Source: CAD feature listing. Evaluate the final solid. Frame: model axes, mm. A direction names the side the tool comes from. Round coordinates to 2 decimals unless told otherwise and drop trailing zeros. Loops run counter-clockwise (first coordinate to the right, second up) from the corner with the lowest first, then second, coordinate; pieces in that order, holes last. Notation, with made-up numbers: (55.5, -3) - (113.5, -3) arc R18 ccw to (113.5, 29) - close; hole circle Ø3 at (-19, 65). An arc over 180 degrees is marked (long way). One line per question, with ' | ' between items. Start each with the question number.
1. Mould query, pull axis Z, two halves, no side actions, for faces 1 (the cylindrical face through (28.14, 71.59, -8.86)), 2 (the flat face through (27.41, 65, 11.34)), 3 (the flat face through (26, 63.5, 11)). Classes: pulls with the +Z half, pulls with the -Z half, needs draft (parallel to the pull), parting line crosses it, or undercut.
2. Pin query (flat end, axial travel): pin 1 (1.5 mm diameter, centred on x = 13, y = 61, fed in from +Z); pin 2 (6 mm diameter, centred on x = -11.5, y = 41.5, fed in from +Z); pin 3 (8 mm diameter, centred on x = 1.5, z = 5.5, fed in from +Y). Return the tip coordinate at first contact, or that it passes through.
3. Cut plane C-C (z = 0). Return loops of the section in (x, y), then the cut area to 3 significant figures.
4. Access query for faces 4 (the cylindrical face through (28.14, 32.07, 8.86)), 5 (the cylindrical face through (25.865, 70.648, -10.724)), 6 (the cylindrical face through (-4.036, 32.955, -30.736)). Directions: +Z, -Z, +X, -X, +Y, -Y. A direction counts if a zero-diameter tool reaches every point of the face in a straight line with its end or side. Return the directions, or none.
5. Ray query, line 1 (Y direction, x = 3, z = -28); line 2 (X direction, y = 30, z = 0). Return the intervals inside material, ascending.
6. Cut plane A-A (y = 12). Return loops of the section in (x, z).
7. Cut plane B-B (x = 0). Return loops of the section in (y, z), then the cut area to 3 significant figures.
Autodesk Inventor part; units mm, degrees
ref_plane "YZ Plane" through (0, 0, 0) normal (1, 0, 0) x (0, 1, 0)
ref_plane "XZ Plane" through (0, 0, 0) normal (0, 1, 0) x (-1, 0, 0)
ref_plane "XY Plane" through (0, 0, 0) normal (0, 0, 1) x (1, 0, 0)
sketch "Sketch1" plane through (0, 0, 0) normal (0, 0, 1) x (1, 0, 0)
  line L0 (0, 0) -> (31, 0)
  line L1 (31, 0) -> (31, 65)
  line L2 (31, 65) -> (29.5, 65)
  line L3 (29.5, 65) -> (29.5, 78)
  line L4 (29.5, 78) -> (28, 78)
  line L5 (28, 76.5) -> (28, 76.5)
  line L6 (28, 78) -> (28, 63.5)
  line L7 (28, 63.5) -> (29.5, 63.5)
  line L8 (29.5, 63.5) -> (29.5, 1.5)
  line L9 (29.5, 1.5) -> (0, 1.5)
  line L10 (0, 0) -> (0, 76.5) construction
  line L11 (0, 0) -> (0, 1.5)
  dimension "d1" = 31
  dimension "d2" = 65
  dimension "d3" = 1.5
  dimension "d4" = 13
  dimension "d5" = 1.5
  dimension "d6" = 1.5
revolve "Revolution1" add sketch "Sketch1" angle 360 about axis through (0, 0, 0) along (0, 1, 0)
properties part number "yellow_base"
Answers follow:
1) face 1: parting line crosses it | face 2: needs draft | face 3: undercut
2) pin 1: stops at z = 28.48 | pin 2: stops at z = 29.81 | pin 3: stops at y = 1.5
3) outline: (-31, 0) - (31, 0) - (31, 65) - (29.5, 65) - (29.5, 78) - (28, 78) - (28, 63.5) - (29.5, 63.5) - (29.5, 1.5) - (-29.5, 1.5) - (-29.5, 63.5) - (-28, 63.5) - (-28, 78) - (-29.5, 78) - (-29.5, 65) - (-31, 65) - close | area: 327 mm2
4) face 4: none | face 5: +Y | face 6: +Y, -Y
5) line 1: y = 0 to 1.5, 63.5 to 78 | line 2: x = -31 to -29.5, 29.5 to 31
6) outline: circle Ø62 at (0, 0); hole circle Ø59 at (0, 0)
7) outline: (0, -31) - (65, -31) - (65, -29.5) - (78, -29.5) - (78, -28) - (63.5, -28) - (63.5, -29.5) - (1.5, -29.5) - (1.5, 29.5) - (63.5, 29.5) - (63.5, 28) - (78, 28) - (78, 29.5) - (65, 29.5) - (65, 31) - (0, 31) - close | area: 327 mm2
